Study the drawing (mm; zero at the part's minimum x, y, z) and answer. A direction names the side the tool comes from. Coordinates: 2 decimals unless noted, no trailing zeros. Order: outer loops, then holes, each group sorted by start corner. A loop starts at its lowest first (then second) coordinate and runs counter-clockwise, first axis right, second up. Notation, with made-up numbers: M -19.75,66 L 30.25,66 A13 ccw 30.25,90 Z; hole C -38.5,44 d1. An arc over 180 degrees is marked long. Put each result on its own line as item: value.
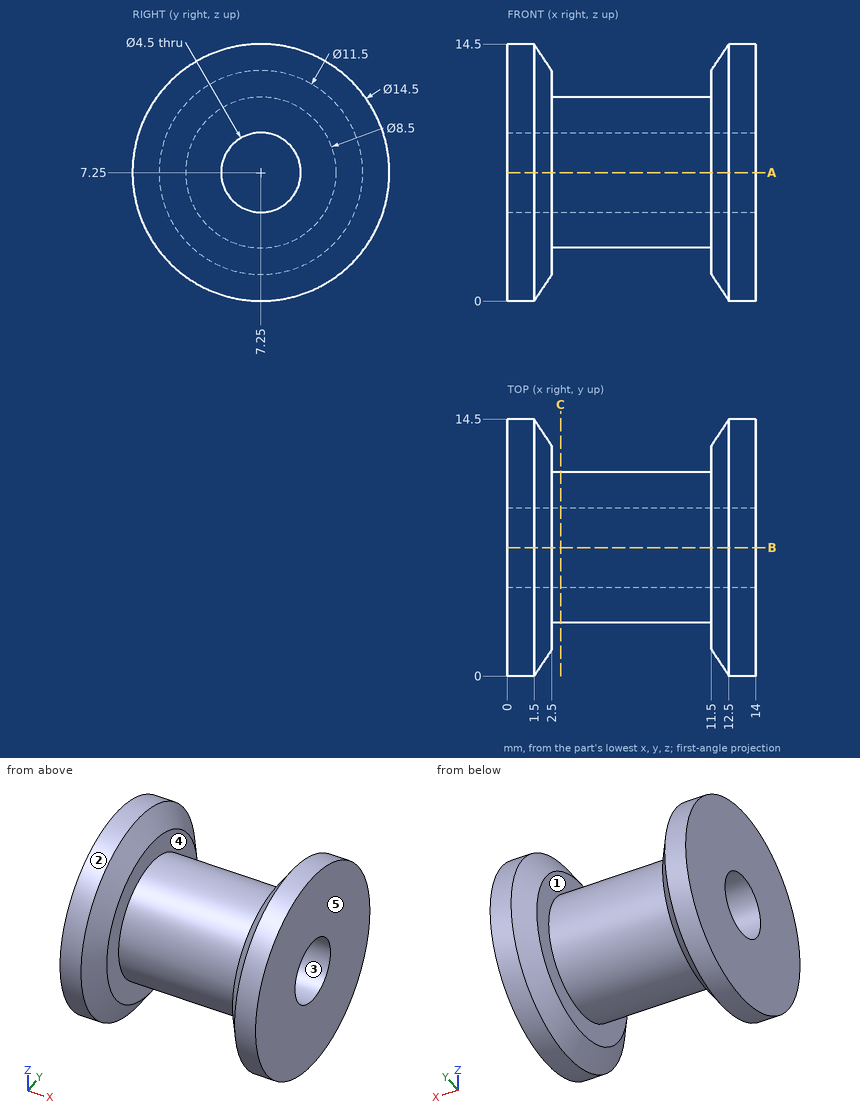
Q1. Find section C-C on x = 3. Write down the section's boundary in (y, z), plus the area to 3 significant figures.
Answers below:
outline: C 7.25,7.25 d8.5; hole C 7.25,7.25 d4.5
area: 40.8 mm^2
Q2. Consider line 1 along X through (y, z) = (10.75, 2.75); line 2 along Z through (x, y) = (10.25, 7.25); line 3 along Y through (x, z) = (7, 6.5). Determine where each line is inside the solid, lowest interval first.
Answers below:
line 1: x = 0 to 2.5, 11.5 to 14
line 2: z = 3 to 5, 9.5 to 11.5
line 3: y = 3.07 to 5.13, 9.37 to 11.43
Q3. Given pin 1 (2 mm diameter, centred on x = 7.5, z = 13, fed in from -Y); pin 2 (1.5 mm diameter, centred on x = 2, z = 4, fed in from +Y), each flat-ended and moving along its own axis, determine where each tip first touches the part or whether it passes through.
Answers below:
pin 1: passes through
pin 2: stops at y = 13.98
Q4. Find section A-A on z = 7.25. Write down the section's boundary in (x, y), plus the area to 3 significant figures.
Answers below:
outline: M 0,0 L 1.5,0 L 2.5,1.5 L 2.5,3 L 11.5,3 L 11.5,1.5 L 12.5,0 L 14,0 L 14,5 L 0,5 Z; M 0,9.5 L 14,9.5 L 14,14.5 L 12.5,14.5 L 11.5,13 L 11.5,11.5 L 2.5,11.5 L 2.5,13 L 1.5,14.5 L 0,14.5 Z
area: 83.0 mm^2
Q5. A tool of negligible diameter and unlimited length cuts with its end or side. For the marked faces 1 and 2, from which of +Z, -Z, +X, -X, +Y, -Y can it reach the whole face along a straight path? Write none if from no direction.
Answers below:
face 1: none
face 2: +X, -X
Q6. For a pull along X with two mould halves and no side action, classify the marked faces 3, 4 and 5 as +X half, -X half, draft (parallel to the pull), parting line (faces both ways), or undercut.
Answers below:
face 3: draft
face 4: undercut
face 5: +X half
